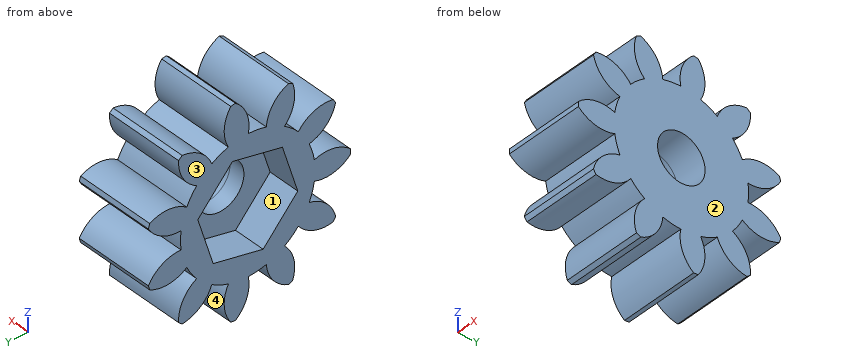
```python
from build123d import *

# Parameters (mm, degrees)
BASPROSKE_W             = 5
BASPROSKE_H             = 6.5
TOOTHCUT_DEPTH          = 11.464224768
TEETHCUTS_COUNT         = 11
TEETHCUTS_ANGLE         = 327.272727273
BORSKE_R                = 1.5
BORE_DEPTH              = 50.0000508
ESQUISSE1_R             = 2.75
ENL_V_MAT_EXTRU_1_DEPTH = 3
ESQUISSE2_R             = 2.75
ESQUISSE2_R_2           = 1.5
BOSS_EXTRU_1_DEPTH      = 3
ENL_V_MAT_EXTRU_2_DEPTH = 2


with BuildPart() as part:
    # BasProSke → Base-Revolve (revolve)
    with BuildSketch(Plane(origin=(0, 0, 0), x_dir=(1, 0, 0), z_dir=(0, 1, 0)), mode=Mode.PRIVATE) as base_revolve_sk:
        with Locations((2.5, 3.25)):
            Rectangle(BASPROSKE_W, BASPROSKE_H)
    revolve(base_revolve_sk.sketch.rotate(Axis((-10, 0, 0), (1, 0, 0)), 180), axis=Axis((-10, 0, 0), (1, 0, 0)))

    # TooCutSke → ToothCut (cut, through all)
    with BuildSketch(Plane(origin=(0, 0, 0), x_dir=(0, 0, -1), z_dir=(1, 0, 0))):
        with BuildLine():
            ThreePointArc((0.576045815, 4.209771041), (0, 4.249), (-0.576045815, 4.209771041))
            ThreePointArc((-0.576045815, 4.209771041), (-0.841371334, 5.420048739), (-1.718652745, 6.295004202))
            ThreePointArc((-1.718652745, 6.295004202), (0, 6.5254), (1.718652745, 6.295004202))
            ThreePointArc((1.718652745, 6.295004202), (0.841371334, 5.420048739), (0.576045815, 4.209771041))
        make_face()
    toothcut = extrude(amount=TOOTHCUT_DEPTH, mode=Mode.SUBTRACT)

    # TeethCuts: ToothCut ×11 about axis
    teethcuts_axis = Axis((-10, 0, 0), (1, 0, 0))
    for i in range(1, TEETHCUTS_COUNT):
        add(toothcut.rotate(teethcuts_axis, i * TEETHCUTS_ANGLE / (TEETHCUTS_COUNT - 1)), mode=Mode.SUBTRACT)

    # BorSke → Bore (cut, symmetric)
    with BuildSketch(Plane(origin=(0, 0, 0), x_dir=(0, 0, -1), z_dir=(1, 0, 0))):
        with Locations(Location((0, 0, 0), (0, 0, 180))):
            Circle(BORSKE_R)
    extrude(amount=BORE_DEPTH, both=True, mode=Mode.SUBTRACT)

    # Esquisse1 → Enlèv. mat.-Extru.1 (cut)
    with BuildSketch(Plane.ZY):
        Circle(ESQUISSE1_R)
    extrude(amount=-ENL_V_MAT_EXTRU_1_DEPTH, mode=Mode.SUBTRACT)

    # Esquisse2 → Boss.-Extru.1 (add)
    with BuildSketch(Plane.ZY.offset(-3)):
        Circle(ESQUISSE2_R)
        Circle(ESQUISSE2_R_2, mode=Mode.SUBTRACT)
    extrude(amount=BOSS_EXTRU_1_DEPTH)

    # Esquisse3 → Enlèv. mat.-Extru.2 (cut)
    with BuildSketch(Plane.ZY):
        Polygon((2.381429268, -2.186807713), (3.084545667, 0.968974387), (0.703116398, 3.1557821), (-2.381429268, 2.186807713), (-3.084545667, -0.968974387), (-0.703116398, -3.1557821), align=None)
    extrude(amount=-ENL_V_MAT_EXTRU_2_DEPTH, mode=Mode.SUBTRACT)


solid = part.part
```
Verification items for the finished model (mm, model axes). Face numbers are marked on the shaded views. A direction names the side the tool comes from. Coordinates: 2 decimals unless noted, no trailing zeros. Loops run counter-clockwise (first coordinate to the right, second up) from the corner with the lowest first, then second, coordinate; pieces in that order, holes last. Notation, with made-up numbers: (60, 67.5) - (82, 67.5) arc R16 ccw to (82, 92.5) - close; hole circle Ø4 at (59.25, 72). An arc over 180 degrees is marked (long way). Return JSON: item names as keys, results as strings.
1. Tool access check on the marked faces 1 and 2. Record the directions out of +Z, -Z, +X, -X, +Y, -Y that give a thin tool (end or side, any length) a straight path to the whole face; none if there is none.
Established:
{"face 1": "-X", "face 2": "+Z, -Z, +X, +Y, -Y"}
2. Go/stop test with flat-tipped pins: pin 1 (1 mm diameter, centred on x = 1.5, z = 4.5, fed in from +Y); pin 2 (2 mm diameter, centred on x = 3.5, y = -3, fed in from -Z). Record where each tip stops, or that it passes through.
Established:
{"pin 1": "stops at y = 4.37", "pin 2": "stops at z = -5.97"}
3. Section check A-A, the plane y = -5. Record the boundary of the cut face in (x, z).
Established:
{"outline": "(0, -3.68) - (5, -3.68) - (5, -2.37) - (0, -2.37) - close; (0, -0.77) - (5, -0.77) - (5, 0.77) - (0, 0.77) - close; (0, 2.37) - (5, 2.37) - (5, 3.68) - (0, 3.68) - close"}
4. Mould release check, pull along Z, two halves, no side actions. Record for the marked faces 3 and 4: +Z half, -Z half, draft (parallel to the pull), parting line (faces both ways), or undercut.
Established:
{"face 3": "draft", "face 4": "undercut"}
5. Section check B-B, the plane z = -1. Record the boundary of the cut face in (x, y).
Established:
{"outline": "(0, -4.13) - (5, -4.13) - (5, -1.12) - (2, -1.12) - (2, -2.88) - (0, -2.88) - close; (0, 2.62) - (2, 2.62) - (2, 1.12) - (5, 1.12) - (5, 5.67) - (0, 5.67) - close"}
6. Thickness scan on L1, parallel to Y at x = 1.1, z = -4.75; L2, parallel to Y at x = 3.15, z = 1.25; L3, parallel to Y at x = 1.65, z = -0.5. Record the ranges inside material, lowest first.
Established:
{"L1": "y = -2.93 to -1.32, -0.08 to 1.46, 3.28 to 4.37", "L2": "y = -4.06 to -0.83, 0.83 to 5.95", "L3": "y = -6.02 to -3.09, 2.78 to 4.22"}
